Source: CAD feature listing. Evaluate the final solid. Frame: model axes, mm. A direction names the side the tool comes from. Coordinates: 2 decimals unless noted, no trailing zeros. Order: outer loops, then holes, each group sorted by start corner. A loop starts at its lowest first (then second) coordinate and runs counter-clockwise, first axis right, second up. Notation, with made-up numbers: (45, 71) -> (102, 71) arc R37 cw to (102, 110) -> close; hole circle Ø11 at (84.25, 50.25). An arc over 180 degrees is marked (long way). Put each result on its own line as item: value.
from build123d import *

# Parameters (mm, degrees)
F1_DEPTH = 15
F2_R     = 3
F3_DEPTH = 10


with BuildPart() as f1:
    # F0 (on Right) → F1 (new body)
    with BuildSketch(Plane.YZ):
        with BuildLine():
            Line((15.411535, 0), (-15.411535, 0))
            Line((-15.411535, 0), (-15.411535, -10.5))
            ThreePointArc((-15.411535, -10.5), (-22.911535, -18), (-30.411535, -10.5))
            ThreePointArc((-30.411535, -10.5), (-32.911535, -8), (-35.411535, -10.5))
            ThreePointArc((-35.411535, -10.5), (-24.532361, -22.894471), (-10.831867, -13.714286))
            ThreePointArc((-10.831867, -13.714286), (-9.047247, -11.035875), (-6, -10))
            Line((-6, -10), (6, -10))
            ThreePointArc((6, -10), (9.047247, -11.035875), (10.831867, -13.714286))
            ThreePointArc((10.831867, -13.714286), (24.532361, -22.894471), (35.411535, -10.5))
            ThreePointArc((35.411535, -10.5), (32.911535, -8), (30.411535, -10.5))
            ThreePointArc((30.411535, -10.5), (22.911535, -18), (15.411535, -10.5))
            Line((15.411535, -10.5), (15.411535, 0))
        make_face()
    extrude(amount=F1_DEPTH)

    # F2 (on face) → F3 (cut, through all)
    with BuildSketch(Plane(origin=(0, 0, -10), x_dir=(1, 0, 0), z_dir=(0, 0, -1))):
        with Locations((7.5, 0)):
            Circle(F2_R)
    extrude(amount=-F3_DEPTH, mode=Mode.SUBTRACT)


solid = f1.part
1. Pull-direction query (X, two-part tool) for faces 1 (the cylindrical face through (10.27, 1.15, -5.07)), 2 (the flat face through (15, 0, -9)), 3 (the flat face through (0, 0, -9)), 4 (the flat face through (9, 3, -10)); classes: pulls with the +X half, pulls with the -X half, needs draft (parallel to the pull), parting line crosses it, or undercut.
Numbers:
face 1: undercut
face 2: pulls with the +X half
face 3: pulls with the -X half
face 4: needs draft
2. Cut plane A-A on y = 0. Output: boundary loops of the cut face in (x, z), plus the area to 3 significant figures.
Numbers:
outline: (0, -10) -> (4.5, -10) -> (4.5, 0) -> (0, 0) -> close; (10.5, -10) -> (15, -10) -> (15, 0) -> (10.5, 0) -> close
area: 90.0 mm2
3. Ray query, line 1 along Y through (x, z) = (4.25, -20.5); line 2 along Y through (x, z) = (7.5, -4.5); line 3 along X through (y, z) = (0, -3.75). Return the intervals inside material, ascending.
Numbers:
line 1: y = -30.41 to -15.41, 15.41 to 30.41
line 2: y = -15.41 to -3, 3 to 15.41
line 3: x = 0 to 4.5, 10.5 to 15
4. Cut plane D-D on z = -11.75. Output: boundary loops of the cut face in (x, y), plus the area to 3 significant figures.
Numbers:
outline: (0, -35.35) -> (15, -35.35) -> (15, -30.31) -> (0, -30.31) -> close; (0, -15.52) -> (15, -15.52) -> (15, -9.8) -> (0, -9.8) -> close; (0, 9.8) -> (15, 9.8) -> (15, 15.52) -> (0, 15.52) -> close; (0, 30.31) -> (15, 30.31) -> (15, 35.35) -> (0, 35.35) -> close
area: 323 mm2
5. Cut plane C-C on x = 7.5. Output: boundary loops of the cut face in (y, z).
Numbers:
outline: (-35.41, -10.5) arc R12.5 ccw to (-10.83, -13.71) arc R5 cw to (-6, -10) -> (-3, -10) -> (-3, 0) -> (-15.41, 0) -> (-15.41, -10.5) arc R7.5 cw to (-30.41, -10.5) arc R2.5 ccw to start; (3, -10) -> (6, -10) arc R5 cw to (10.83, -13.71) arc R12.5 ccw to (35.41, -10.5) arc R2.5 ccw to (30.41, -10.5) arc R7.5 cw to (15.41, -10.5) -> (15.41, 0) -> (3, 0) -> close
6. Cut plane B-B on z = -20.5. Output: boundary loops of the cut face in (x, y).
Numbers:
outline: (0, -30.41) -> (15, -30.41) -> (15, -15.41) -> (0, -15.41) -> close; (0, 15.41) -> (15, 15.41) -> (15, 30.41) -> (0, 30.41) -> close
7. First-contact query: pin 1 (4 mm diameter, centred on x = 4.5, z = -7, fed in from -Y); pin 2 (4 mm diameter, centred on x = 8, y = 18, fed in from -Z); pin 3 (5 mm diameter, centred on x = 7.5, y = 0, fed in from -Z); pin 4 (3 mm diameter, centred on x = 13.5, z = -6, fed in from +Y). Flat tips, straight axial feed; report the tip coordinate or a pass-through.
Numbers:
pin 1: stops at y = -34.91
pin 2: stops at z = -22.66
pin 3: passes through
pin 4: stops at y = 15.41
8. Set-up query: faces 5 (the cylindrical face through (7, 9, -11)), 6 (the flat face through (4, 0, 0)), 7 (the flat face through (7, 15.412, -5)). Return all of +Z, -Z, +X, -X, +Y, -Y with unobstructed straight access to the full face (end or side cutting, diameter ignored); none if empty.
Numbers:
face 5: -Z, +X, -X
face 6: +Z, +X, -X, +Y, -Y
face 7: +Z, +X, -X
